Geometry check sheet. Reference: the model listing, model coordinates, mm. A direction names the side the tool comes from. Round coordinates to 2 decimals unless told otherwise and drop trailing zeros. Order: outer loops, then holes, each group sorted by start corner. A loop starts at its lowest first (then second) coordinate and runs counter-clockwise, first axis right, second up. Notation, with made-up numbers: M 60,34.5 L 82,34.5 A20 cw 82,57.5 Z; hole C 31.5,69 d6. An arc over 180 degrees is marked long. Return JSON: item names as keys, results as strings. Group by question number.
```python
from build123d import *

# Parameters (mm, degrees)
F2_R      = 68
F3_DEPTH  = 500
F1_FACE_R = 68.2
F4_DEPTH  = 200


with BuildPart() as f1:
    # F0 (on Front) → F1 (revolve)
    with BuildSketch(Plane.XZ):
        Polygon((-249.4, 165.3), (-114, 165.3), (0, 165.3), (0, 367.3), (-68.2, 367.3), (-68.2, 245), (-74.2, 245), (-74.2, 367.3), (-249.4, 367.3), align=None)
    revolve(axis=Axis((0, 0, 266.3), (0, 0, -1)))

    # F2 (on Front) → F3 (join)
    with BuildSketch(Plane.XZ):
        with Locations((-181.4, 270)):
            Circle(F2_R)
    extrude(amount=F3_DEPTH)

    # F1_face (on face) → F4 (join)
    with BuildSketch(Plane.XY.offset(367.3)):
        Circle(F1_FACE_R)
    extrude(amount=F4_DEPTH)


solid = f1.part
```
Q1. Set-up check for faces 1 (the face through (-1, 1, 567.3)), 2 (the face through (9.66, 73.57, 307.01)), 3 (the face through (-249.334, -302.056, 272.99)): record each of +Z, -Z, +X, -X, +Y, -Y from which the full face is reachable in a straight line by a thin tool's end or side.
Q2. Section check D-D on z = 394. Record the cut outline in (x, y), plus the area to 3 significant figures.
Q3. Material ranges on line 1 along Y through (x, z) = (0, 275); line 2 along Z through (x, y) = (-184, -459); line 3 along Z through (x, y) = (-184, 48), recorded low to high.
Q4. Release check for a two-part mould opening along Y. For faces 4 (the face through (3, 3, 165.3)), 5 (the face through (33, -60, 245)), 6 (the face through (-182, -500, 271)) record: +Y half, -Y half, draft (parallel to the pull), parting line (faces both ways), or undercut.
Q5. Depth check by flat-ended pin: pin 1 Ø3 at (y, z) = (3, 476.5) entering from -X; pin 2 Ø8 at (y, z) = (59, 244.5) entering from -X; pin 3 Ø12 at (x, y) = (145, -83) entering from +Z. Enter the tip coordinate at first touch or a pass-through.
Q6. Section check A-A on x = 0. Record the cut outline in (y, z).
Q7. Section check B-B on z = 291. Record the cut outline in (x, y).
Q8. Section check C-C on y = -25. Record the cut outline in (x, z).
Geometry check:
{
 "1": {"face 1": "+Z, +X, -X, +Y, -Y", "face 2": "+Z", "face 3": "-Y"},
 "2": {"outline": "C 0,0 d136.4", "area": "14,600 mm^2"},
 "3": {"line 1": "y = -249.4 to -74.2, -68.2 to 68.2, 74.2 to 249.4", "line 2": "z = 202.05 to 337.95", "line 3": "z = 165.3 to 367.3"},
 "4": {"face 4": "draft", "face 5": "undercut", "face 6": "-Y half"},
 "5": {"pin 1": "stops at x = -68.18", "pin 2": "stops at x = -243.26", "pin 3": "stops at z = 367.3"},
 "6": {"outline": "M -249.4,165.3 L 249.4,165.3 L 249.4,367.3 L 74.2,367.3 L 74.2,245 L 68.2,245 L 68.2,567.3 L -68.2,567.3 L -68.2,245 L -74.2,245 L -74.2,367.3 L -249.4,367.3 Z"},
 "7": {"outline": "M -246.08,-500 L -116.72,-500 L -116.72,-220.4 A249.4 ccw long -246.08,-40.58 Z; C 0,0 d136.4; hole C 0,0 d148.4"},
 "8": {"outline": "M -248.14,165.3 L 248.14,165.3 L 248.14,367.3 L 69.86,367.3 L 69.86,245 L 63.45,245 L 63.45,567.3 L -63.45,567.3 L -63.45,245 L -69.86,245 L -69.86,367.3 L -248.14,367.3 L -248.14,283.01 A68 ccw -248.14,256.99 Z"}
}
